The model under review builds one solid part; all positions refer to its coordinate system, in mm. A direction names the side the tool comes from. Give positions to 0.01 mm unless a question says otherwise; leave off trailing zeros. Order: outer loops, then holes, each group sorted by start corner. A loop starts at its lowest first (then second) coordinate and runs counter-clockwise, first axis right, second up. Notation, with made-up numbers: (1.5, -10.75) - (16.5, -10.75) arc R23 ccw to (16.5, 26.25) - close; hole circle Ø2 at (-29, 14.5). An arc over 180 degrees is marked (long way). Put each result on its own line as item: value.
```python
from build123d import *

# Parameters (mm, degrees)
EXTRUDE_1_DEPTH     = 250
SKETCH_2_R          = 2.5
EXTRUDE_2_DEPTH     = 10
SKETCH_3_R          = 5
EXTRUDE_3_DEPTH     = 10
SKETCH_4_W          = 2
SKETCH_4_H          = 1.835573614
CUT_EXTRUDE_1_DEPTH = 10
EXTRUDE_START       = -5
SKETCH_6_R          = 2.5
EXTRUDE_5_DEPTH     = 5
SKETCH_9_R          = 2.5
EXTRUDE_7_DEPTH     = 5
SKETCH_10_R         = 2.5
CUT_EXTRUDE_3_DEPTH = 3
CUT_EXTRUDE_START   = -3
SKETCH_11_R         = 2.5
CUT_EXTRUDE_4_DEPTH = 3
EXTRUDE_START_2     = -10
SKETCH_12_R         = 5
EXTRUDE_8_DEPTH     = 10
SKETCH_14_R         = 2.5
EXTRUDE_10_DEPTH    = 1
SKETCH_15_W         = 12
SKETCH_15_H         = 12
EXTRUDE_11_DEPTH    = 250
SKETCH_16_R         = 4
EXTRUDE_12_DEPTH    = 20


with BuildPart() as part:
    # 草图1 → 凸台-拉伸1 (new body)
    with BuildSketch(Plane.XY):
        Polygon((5, 0), (2.5, 4.330127019), (-2.5, 4.330127019), (-5, 0), (-2.5, -4.330127019), (2.5, -4.330127019), align=None)
    extrude(amount=EXTRUDE_1_DEPTH)

    # 草图2 → 凸台-拉伸2 (add)
    with BuildSketch(Plane.XY.offset(250)):
        Circle(SKETCH_2_R)
    extrude(amount=EXTRUDE_2_DEPTH)

    # 草图3 → 凸台-拉伸3 (add)
    with BuildSketch(Plane(origin=(0, 0, 0), x_dir=(-1, 0, 0), z_dir=(0, 0, -1))):
        Circle(SKETCH_3_R)
    extrude(amount=EXTRUDE_3_DEPTH)

    # 草图4 → 切除-拉伸1 (cut)
    with BuildSketch(Plane.XY.offset(260)):
        with Locations((0, 2.417786807)):
            Rectangle(SKETCH_4_W, SKETCH_4_H)
    extrude(amount=-CUT_EXTRUDE_1_DEPTH, mode=Mode.SUBTRACT)

    # 草图6 → 凸台-拉伸5 (add)
    with BuildSketch(Plane.XY.offset(260).offset(EXTRUDE_START)):
        with Locations(Location((0, 0, 0), (0, 0, 113.578178478))):
            Circle(SKETCH_6_R)
    extrude(amount=EXTRUDE_5_DEPTH)

    # 草图9 → 凸台-拉伸7 (add)
    with BuildSketch(Plane(origin=(0, 0, -10), x_dir=(-1, 0, 0), z_dir=(0, 0, -1))):
        with Locations(Location((0, 0, 0), (0, 0, 66.421821522))):
            Circle(SKETCH_9_R)
    extrude(amount=-EXTRUDE_7_DEPTH)

    # 草图10 → 切除-拉伸3 (cut)
    with BuildSketch(Plane(origin=(0, 0, -10), x_dir=(-1, 0, 0), z_dir=(0, 0, -1))):
        with Locations(Location((0, 0, 0), (0, 0, 66.421821522))):
            Circle(SKETCH_10_R)
    extrude(amount=-CUT_EXTRUDE_3_DEPTH, mode=Mode.SUBTRACT)

    # 草图11 → 切除-拉伸4 (cut)
    with BuildSketch(Plane.XY.offset(260).offset(CUT_EXTRUDE_START)):
        with Locations(Location((0, 0, 0), (0, 0, 113.578178478))):
            Circle(SKETCH_11_R)
    extrude(amount=CUT_EXTRUDE_4_DEPTH, mode=Mode.SUBTRACT)

    # 草图12 → 凸台-拉伸8 (add)
    with BuildSketch(Plane(origin=(0, 0, -10), x_dir=(-1, 0, 0), z_dir=(0, 0, -1)).offset(EXTRUDE_START_2)):
        Circle(SKETCH_12_R)
    extrude(amount=EXTRUDE_8_DEPTH)

    # 草图14 → 凸台-拉伸10 (add)
    with BuildSketch(Plane.XY.offset(250)):
        Circle(SKETCH_14_R)
    extrude(amount=EXTRUDE_10_DEPTH)

    # 草图15 → 凸台-拉伸11 (add)
    with BuildSketch(Plane.XY.offset(250)):
        Rectangle(SKETCH_15_W, SKETCH_15_H)
    extrude(amount=-EXTRUDE_11_DEPTH)

    # 草图16 → 凸台-拉伸12 (add)
    with BuildSketch(Plane.XY.offset(257)):
        Circle(SKETCH_16_R)
    extrude(amount=-EXTRUDE_12_DEPTH)


solid = part.part
```
(1) Wall thickness on L1, parallel to Z at x = 3.25, y = -5.5; L2, parallel to Z at x = 3, y = -2.75: over which ranges is each line inside the solid? List them lowest first.
The answers:
L1: 0 to 250
L2: -10 to 250
(2) For faces 1 (the flat face through (0, 6, 127)), 2 (the cylindrical face through (-0.867, -3.905, 253.549)), 3 (the flat face through (5.2, 0.1, 0)), list the 3-axis set-ups (+Z, -Z, +X, -X, +Y, -Y) from which the entire face can be reached by the end or side of a thin tool; tool diameter is ignored.
The answers:
face 1: +Z, -Z, +X, -X, +Y
face 2: +Z
face 3: -Z
(3) Take a section at A-A, the plane x = 1.5. Write out the cut boundary in (y, z), then the cut area to 3 significant figures.
The answers:
outline: (-6, 0) - (-4.77, 0) - (-4.77, -10) - (4.77, -10) - (4.77, 0) - (6, 0) - (6, 250) - (3.71, 250) - (3.71, 257) - (-3.71, 257) - (-3.71, 250) - (-6, 250) - close
area: 3,150 mm^2
